Part model, mm, in its own coordinate system. Face numbers are marked on the shaded views. A direction names the side the tool comes from. Give positions to 0.01 mm unless a question says otherwise; leave off trailing zeros. Write each loop counter-clockwise with the first axis right and the second up, starting at its lowest first coordinate (ties: lowest second). Pieces come first, ordered by that corner, then holes.
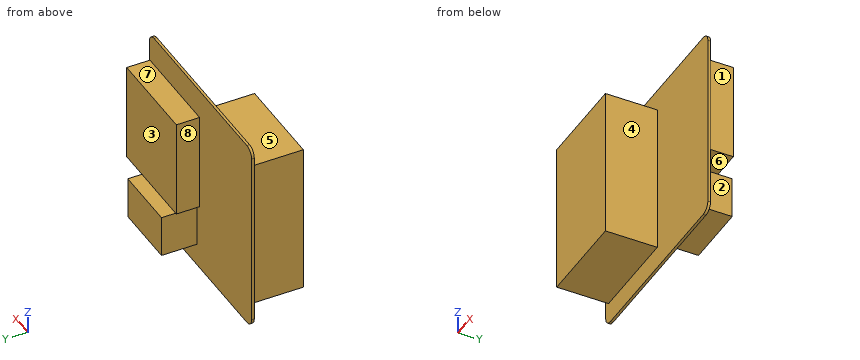
```python
from build123d import *

# Parameters (mm, degrees)
ESQUISSE1_W        = 109
ESQUISSE1_H        = 110
BOSS_EXTRU_1_DEPTH = 1.5
CONG_1_R           = 5
ESQUISSE2_W        = 52
ESQUISSE2_H        = 85.5
BOSS_EXTRU_2_DEPTH = 29
ESQUISSE3_W        = 53
ESQUISSE3_H        = 55.5
ESQUISSE3_W_2      = 50
ESQUISSE3_H_2      = 49
BOSS_EXTRU_3_DEPTH = 13
ESQUISSE4_W        = 50
ESQUISSE4_H        = 49
BOSS_EXTRU_4_DEPTH = 13
ESQUISSE5_W        = 36
ESQUISSE5_H        = 23.5
BOSS_EXTRU_5_DEPTH = 20


with BuildPart() as part:
    # Esquisse1 → Boss.-Extru.1 (new body)
    with BuildSketch(Plane(origin=(0, 0, 0), x_dir=(1, 0, 0), z_dir=(0, 1, 0))):
        with Locations((54.5, 55)):
            Rectangle(ESQUISSE1_W, ESQUISSE1_H)
    extrude(amount=BOSS_EXTRU_1_DEPTH)

    # Congé1
    cong_1_edges = [part.edges().sort_by_distance(p)[0] for p in [
        (0, 0.75, -110),
        (109, 0.75, -110),
        (109, 0.75, 0),
        (0, 0.75, 0),
    ]]
    fillet(cong_1_edges, radius=CONG_1_R)

    # Esquisse2 → Boss.-Extru.2 (add)
    with BuildSketch(Plane.XZ):
        with Locations((29, -54.75)):
            Rectangle(ESQUISSE2_W, ESQUISSE2_H)
    extrude(amount=BOSS_EXTRU_2_DEPTH)

    # Esquisse3 → Boss.-Extru.3 (add)
    with BuildSketch(Plane(origin=(0, 1.5, 0), x_dir=(1, 0, 0), z_dir=(0, 1, 0))):
        with Locations((82, 44.25)):
            Rectangle(ESQUISSE3_W, ESQUISSE3_H)
        with Locations((82, 42.5)):
            Rectangle(ESQUISSE3_W_2, ESQUISSE3_H_2, mode=Mode.SUBTRACT)
    extrude(amount=BOSS_EXTRU_3_DEPTH)

    # Esquisse4 → Boss.-Extru.4 (add)
    with BuildSketch(Plane(origin=(0, 1.5, 0), x_dir=(1, 0, 0), z_dir=(0, 1, 0))):
        with Locations((82, 42.5)):
            Rectangle(ESQUISSE4_W, ESQUISSE4_H)
    extrude(amount=BOSS_EXTRU_4_DEPTH)

    # Esquisse5 → Boss.-Extru.5 (add)
    with BuildSketch(Plane(origin=(0, 1.5, 0), x_dir=(1, 0, 0), z_dir=(0, 1, 0))):
        with Locations((76, 85.25)):
            Rectangle(ESQUISSE5_W, ESQUISSE5_H)
    extrude(amount=BOSS_EXTRU_5_DEPTH)


solid = part.part
```
1) 3-axis set-ups, long thin cutter, end or side, ignore diameter. For the marked faces 1, 2, 3, 4 and 5: which of +Z, -Z, +X, -X, +Y, -Y reach the whole face in a straight line?
Answers follow:
face 1: +Z, -Z, +X, +Y
face 2: -Z, +X, +Y
face 3: +Z, +X, -X, +Y
face 4: +Z, -Z, +X, -Y
face 5: +Z, +X, -X, -Y
2) Saw through at C-C, the plane x = 28.5. Write the cut outline in (y, z), then the cut area to 3 significant figures.
Answers follow:
outline: (-29, -97.5) - (0, -97.5) - (0, -110) - (1.5, -110) - (1.5, 0) - (0, 0) - (0, -12) - (-29, -12) - close
area: 2,640 mm2
3) Saw through at A-A, the plane y = 11. Write the cut outline in (x, z), then the cut area to 3 significant figures.
Answers follow:
outline: (55.5, -72) - (108.5, -72) - (108.5, -16.5) - (55.5, -16.5) - close; (58, -97) - (94, -97) - (94, -73.5) - (58, -73.5) - close
area: 3,790 mm2
4) Wall check: L1, parallel to Z at x = 66.5, y = 11; L2, parallel to Y at x = 95, z = -57.5; L3, parallel to Y at x = 53, z = -47. Give the ranges that are in metal, low to high.
Answers follow:
L1: z = -97 to -73.5, -72 to -16.5
L2: y = 0 to 14.5
L3: y = -29 to 1.5
5) Saw through at B-B, the plane z = -70. Write the cut outline in (x, y).
Answers follow:
outline: (0, 0) - (3, 0) - (3, -29) - (55, -29) - (55, 0) - (109, 0) - (109, 1.5) - (108.5, 1.5) - (108.5, 14.5) - (55.5, 14.5) - (55.5, 1.5) - (0, 1.5) - close
6) Two-plate mould, pull along Z, no slides. Class the marked faces 6, 7 and 8: +Z half, -Z half, draft (parallel to the pull), parting line (faces both ways), or undercut.
Answers follow:
face 6: undercut
face 7: +Z half
face 8: draft
7) Pin check, flat tips, straight feed: pin 1 Ø6 at (y, z) = (13.5, -85) entering from +X; pin 2 Ø23 at (y, z) = (-15, -69) entering from +X; pin 3 Ø22 at (y, z) = (16.5, -84) entering from -X; pin 4 Ø10 at (x, y) = (36.5, 11) entering from +Z. Stop position of each tip, or through.
Answers follow:
pin 1: stops at x = 94
pin 2: stops at x = 55
pin 3: stops at x = 58
pin 4: passes through
8) Saw through at D-D, the plane y = -9. Write the cut outline in (x, z).
Answers follow:
outline: (3, -97.5) - (55, -97.5) - (55, -12) - (3, -12) - close
